Could you check a few things on this model? Use its own coordinates, in mm. A direction names the side the tool comes from. Give positions to 0.01 mm unless a question says otherwise; leave off trailing zeros. Order: outer loops, then holes, each group sorted by start corner. A loop starts at its lowest first (then second) coordinate and runs counter-clockwise, first axis right, second up. Notation, with made-up numbers: (-2, -24.75) - (21, -24.75) arc R30 cw to (21, 2.25) - close; hole circle Ø10 at (64, 76.5). An arc over 180 degrees is marked (long way). Put each result on its own line as item: value.
from build123d import *

# Parameters (mm, degrees)
SKETCH1_W               = 96.89
SKETCH1_H               = 90.17
PCB_DEPTH               = 1.57
SKETCH2_R               = 2
M3_MOUNTING_HOLES_DEPTH = 1.57
SKETCH4_R               = 2
CUT_EXTRUDE1_DEPTH      = 23
BOSS_EXTRUDE2_DEPTH     = 2
BOSS_EXTRUDE3_DEPTH     = 2
SKETCH9_W               = 3
SKETCH9_H               = 19
SKETCH9_W_2             = 7
CUT_EXTRUDE2_DEPTH      = 128.304608561
SKETCH10_W              = 0.5
SKETCH10_H              = 90.17
CUT_EXTRUDE3_DEPTH      = 10
SKETCH11_W              = 60
SKETCH11_H              = 61
CUT_EXTRUDE4_DEPTH      = 10


with BuildPart() as part:
    # Sketch1 → PCB (new body)
    with BuildSketch(Plane(origin=(0, 0, 0), x_dir=(1, 0, 0), z_dir=(0, 1, 0))):
        with Locations((16.200949951, 63.633996534)):
            Rectangle(SKETCH1_W, SKETCH1_H)
    extrude(amount=PCB_DEPTH)

    # Sketch2 → M3 Mounting Holes (cut)
    with BuildSketch(Plane(origin=(0, 1.57, 0), x_dir=(1, 0, 0), z_dir=(0, 1, 0))):
        with Locations(Location((59.565949951, 24.898996534, 0), (0, 0, 270))):
            Circle(SKETCH2_R)
        with Locations(Location((-26.164050049, 27.438996534, 0), (0, 0, 270))):
            Circle(SKETCH2_R)
        with Locations(Location((-26.164050049, 101.098996534, 0), (0, 0, 270))):
            Circle(SKETCH2_R)
        with Locations(Location((59.565949951, 103.638996534, 0), (0, 0, 270))):
            Circle(SKETCH2_R)
    extrude(amount=-M3_MOUNTING_HOLES_DEPTH, mode=Mode.SUBTRACT)

    # Sketch4 → Cut-Extrude1 (cut)
    with BuildSketch(Plane(origin=(0, 1.57, 0), x_dir=(1, 0, 0), z_dir=(0, 1, 0))):
        with Locations(Location((-20.894050049, 88.718996534, 0), (0, 0, 270))):
            Circle(SKETCH4_R)
        with Locations(Location((53.105949951, 88.718996534, 0), (0, 0, 270))):
            Circle(SKETCH4_R)
        with Locations(Location((-20.894050049, 58.718996534, 0), (0, 0, 270))):
            Circle(SKETCH4_R)
        with Locations(Location((53.105949951, 58.718996534, 0), (0, 0, 270))):
            Circle(SKETCH4_R)
    extrude(amount=-CUT_EXTRUDE1_DEPTH, mode=Mode.SUBTRACT)

    # Sketch7 → Boss-Extrude2 (add)
    with BuildSketch(Plane.XY.offset(-45.718996534)):
        Polygon((27.755949951, 1.57), (19.438412086, 15.976398176), (16.073487816, 15.976398176), (7.755949951, 1.57), align=None)
    extrude(amount=BOSS_EXTRUDE2_DEPTH)

    # Sketch8 → Boss-Extrude3 (add)
    with BuildSketch(Plane.XY.offset(-108.718996534)):
        Polygon((27.755949951, 1.57), (19.438412086, 15.976398176), (16.073487816, 15.976398176), (7.755949951, 1.57), align=None)
    extrude(amount=BOSS_EXTRUDE3_DEPTH)

    # Sketch9 → Cut-Extrude2 (cut, through all)
    with BuildSketch(Plane(origin=(0, 1.57, 0), x_dir=(1, 0, 0), z_dir=(0, 1, 0))):
        with Locations((-10.744050049, 28.048996534)):
            Rectangle(SKETCH9_W, SKETCH9_H)
        with Locations((-3.744050049, 28.048996534)):
            Rectangle(SKETCH9_W_2, SKETCH9_H)
        with Locations((3.255949951, 28.048996534)):
            Rectangle(SKETCH9_W, SKETCH9_H)
    extrude(amount=-CUT_EXTRUDE2_DEPTH, mode=Mode.SUBTRACT)

    # Sketch10 → Cut-Extrude3 (cut)
    with BuildSketch(Plane(origin=(0, 1.57, 0), x_dir=(1, 0, 0), z_dir=(0, 1, 0))):
        with Locations((-31.994050049, 63.633996534)):
            Rectangle(SKETCH10_W, SKETCH10_H)
        with Locations((64.395949951, 63.633996534)):
            Rectangle(SKETCH10_W, SKETCH10_H)
    extrude(amount=-CUT_EXTRUDE3_DEPTH, mode=Mode.SUBTRACT)

    # Sketch11 → Cut-Extrude4 (cut)
    with BuildSketch(Plane(origin=(0, 1.57, 0), x_dir=(1, 0, 0), z_dir=(0, 1, 0))):
        with Locations((16.105949951, 76.218996534)):
            Rectangle(SKETCH11_W, SKETCH11_H)
    extrude(amount=-CUT_EXTRUDE4_DEPTH, mode=Mode.SUBTRACT)


solid = part.part
1) I'm going to push flat-ended pins straight in: pin 1 (4.5 mm diameter, centred on x = 59.57, z = -103.64, fed in from +Y); pin 2 (4.5 mm diameter, centred on x = -20.89, z = -88.72, fed in from -Y); pin 3 (4.5 mm diameter, centred on x = 18, y = 7.5, fed in from +Z); pin 4 (0.8 mm diameter, centred on x = -4.5, y = 0.5, fed in from +Z). Where does each tip first touch, or does it pass through?
Filled in:
pin 1: stops at y = 1.57
pin 2: stops at y = 0
pin 3: stops at z = -43.72
pin 4: stops at z = -37.55
2) We'd pull the mould along Z, two halves only. Please class faces 1 (the flat face through (16, 4, -108.719)), 2 (the flat face through (16, 4, -45.719)), 3 (the flat face through (23.655, 8.672, -44.733)): pulls with the +Z half, pulls with the -Z half, needs draft (parallel to the pull), parting line crosses it, or undercut.
Filled in:
face 1: pulls with the -Z half
face 2: undercut
face 3: needs draft
3) Suppose I cut it at A-A, the plane z = -77. List the corners of the cut face in (x, y) for me, and give its area (3 significant figures).
Filled in:
outline: (-31.74, 0) - (-13.89, 0) - (-13.89, 1.57) - (-31.74, 1.57) - close; (46.11, 0) - (64.15, 0) - (64.15, 1.57) - (46.11, 1.57) - close
area: 56.3 mm^2
4) Which directions (+Z, -Z, +X, -X, +Y, -Y) give clear straight access to the entire face, cutting with the end or side of a thin tool? Please do faces 4 (the flat face through (18, 7, -43.719)), 5 (the flat face through (23.655, 8.672, -107.733)), 6 (the flat face through (16, 4, -106.719)).
Filled in:
face 4: +Z, +X, -X, +Y
face 5: +Z, -Z, +X, +Y
face 6: +Y, -Y
5) Suppose I cut it at B-B, the plane x = 40. List the corners of the cut face in (y, z) for me, and give its area (3 significant figures).
Filled in:
outline: (0, -108.72) - (1.57, -108.72) - (1.57, -106.72) - (0, -106.72) - close; (0, -45.72) - (1.57, -45.72) - (1.57, -18.55) - (0, -18.55) - close
area: 45.8 mm^2
6) If I drill on line 1 (Z direction, x = 12, y = 8.75); line 2 (Y direction, x = -17.5, z = -46); line 3 (Z direction, x = 39.5, y = 1.5), over which ranges is the centre line in solid material (lowest first)? Write a range as [from, to].
Filled in:
line 1: z = [-108.72, -106.72], [-45.72, -43.72]
line 2: y = [0, 1.57]
line 3: z = [-108.72, -106.72], [-45.72, -18.55]
7) Suppose I cut it at C-C, the plane z = -28. List the corners of the cut face in (x, y) for me.
Filled in:
outline: (-31.74, 0) - (-28.08, 0) - (-28.08, 1.57) - (-31.74, 1.57) - close; (-24.24, 0) - (-12.24, 0) - (-12.24, 1.57) - (-24.24, 1.57) - close; (-9.24, 0) - (-7.24, 0) - (-7.24, 1.57) - (-9.24, 1.57) - close; (-0.24, 0) - (1.76, 0) - (1.76, 1.57) - (-0.24, 1.57) - close; (4.76, 0) - (64.15, 0) - (64.15, 1.57) - (4.76, 1.57) - close
